Geometry: final body of the model. Coordinates: model frame, mm. Give positions to 0.01 mm unless a question says otherwise; leave off trailing zeros. Loops run counter-clockwise (first coordinate to the right, second up) from the corner with the lowest first, then second, coordinate; pieces in that order, holes last.
from build123d import *

# Parameters (mm, degrees)
F0_W     = 3.175
F0_H     = 17.78
F0_R     = 1.984375
F1_DEPTH = 3.175


with BuildPart() as f1:
    # F0 (on Front) → F1 (new body)
    with BuildSketch(Plane.XZ):
        Polygon((-88.646, -65.532), (-50.546, -65.532), (-50.546, -62.23), (-19.05, -62.23), (-19.05, -65.532), (19.05, -65.532), (19.05, -62.23), (50.546, -62.23), (50.546, -65.532), (88.646, -65.532), (88.646, -62.23), (107.696, -62.23), (196.85, -62.23), (196.85, -44.45), (193.675, -44.45), (193.675, -26.67), (196.85, -26.67), (196.85, -8.89), (193.675, -8.89), (193.675, 8.89), (196.85, 8.89), (196.85, 26.67), (193.675, 26.67), (193.675, 44.45), (196.85, 44.45), (196.85, 62.23), (107.696, 62.23), (88.646, 62.23), (88.646, 65.532), (50.546, 65.532), (50.546, 62.23), (19.05, 62.23), (19.05, 65.532), (-19.05, 65.532), (-19.05, 62.23), (-50.546, 62.23), (-50.546, 65.532), (-88.646, 65.532), (-88.646, 62.23), (-107.696, 62.23), (-196.85, 62.23), (-196.85, 44.45), (-193.675, 44.45), (-193.675, 26.67), (-196.85, 26.67), (-196.85, 8.89), (-193.675, 8.89), (-193.675, -8.89), (-196.85, -8.89), (-196.85, -26.67), (-193.675, -26.67), (-193.675, -44.45), (-196.85, -44.45), (-196.85, -62.23), (-107.696, -62.23), (-88.646, -62.23), align=None)
        with Locations((-106.1085, -35.56)):
            Rectangle(F0_W, F0_H, mode=Mode.SUBTRACT)
        with Locations((-79.121, -52.705)):
            Circle(F0_R, mode=Mode.SUBTRACT)
        with Locations((-66.421, -52.705)):
            Circle(F0_R, mode=Mode.SUBTRACT)
        with Locations((-79.121, -40.005)):
            Circle(F0_R, mode=Mode.SUBTRACT)
        with Locations((-90.2335, -35.56)):
            Rectangle(F0_W, F0_H, mode=Mode.SUBTRACT)
        with Locations((-66.421, -40.005)):
            Circle(F0_R, mode=Mode.SUBTRACT)
        with Locations((66.421, -52.705)):
            Circle(F0_R, mode=Mode.SUBTRACT)
        with Locations((79.121, -52.705)):
            Circle(F0_R, mode=Mode.SUBTRACT)
        with Locations((66.421, -40.005)):
            Circle(F0_R, mode=Mode.SUBTRACT)
        with Locations((79.121, -40.005)):
            Circle(F0_R, mode=Mode.SUBTRACT)
        with Locations((90.2335, -35.56)):
            Rectangle(F0_W, F0_H, mode=Mode.SUBTRACT)
        with Locations((106.1085, -35.56)):
            Rectangle(F0_W, F0_H, mode=Mode.SUBTRACT)
        with Locations((-106.1085, 0)):
            Rectangle(F0_W, F0_H, mode=Mode.SUBTRACT)
        with Locations((-90.2335, 0)):
            Rectangle(F0_W, F0_H, mode=Mode.SUBTRACT)
        with Locations((-106.1085, 35.56)):
            Rectangle(F0_W, F0_H, mode=Mode.SUBTRACT)
        with Locations((-90.2335, 35.56)):
            Rectangle(F0_W, F0_H, mode=Mode.SUBTRACT)
        with Locations((90.2335, 0)):
            Rectangle(F0_W, F0_H, mode=Mode.SUBTRACT)
        with Locations((106.1085, 0)):
            Rectangle(F0_W, F0_H, mode=Mode.SUBTRACT)
        with Locations((90.2335, 35.56)):
            Rectangle(F0_W, F0_H, mode=Mode.SUBTRACT)
        with Locations((106.1085, 35.56)):
            Rectangle(F0_W, F0_H, mode=Mode.SUBTRACT)
    extrude(amount=F1_DEPTH)


solid = f1.part
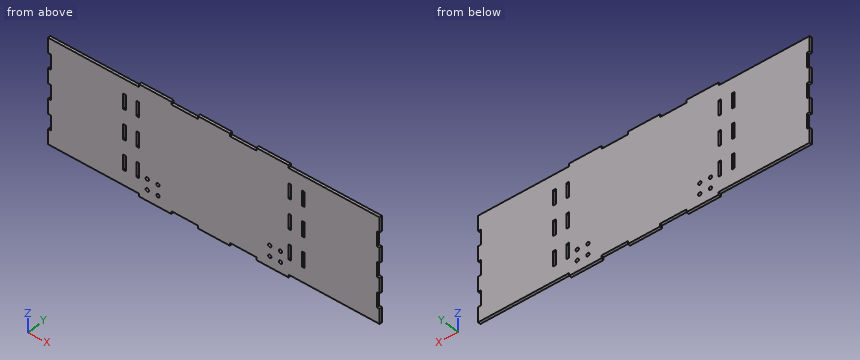
Item 1: Ray query, probe 1 along X at (y, z) = (-2.6, -5.5) (3 decimals); probe 2 along X at (y, z) = (-0.35, -54); probe 3 along Z at (x, y) = (-143.5, -0.2). Return the intervals inside material, ascending.
Values follow:
probe 1: x = -193.675 to -107.696, -104.521 to -91.821, -88.646 to 88.646, 91.821 to 104.521, 107.696 to 193.675
probe 2: x = -196.85 to -80.62, -77.62 to -67.92, -64.92 to 64.92, 67.92 to 77.62, 80.62 to 196.85
probe 3: z = -62.23 to 62.23
Item 2: Section query A-A on z = -1. Return loops of the section in (x, y) (3 decimals).
Values follow:
outline: (-193.675, -3.175) - (-107.696, -3.175) - (-107.696, 0) - (-193.675, 0) - close; (-104.521, -3.175) - (-91.821, -3.175) - (-91.821, 0) - (-104.521, 0) - close; (-88.646, -3.175) - (88.646, -3.175) - (88.646, 0) - (-88.646, 0) - close; (91.821, -3.175) - (104.521, -3.175) - (104.521, 0) - (91.821, 0) - close; (107.696, -3.175) - (193.675, -3.175) - (193.675, 0) - (107.696, 0) - close
Item 3: Section query C-C on y = -0.65. Give the number of separate pieces and of enclosed holes in the cut face, plus the area to 3 significant figures.
Values follow:
separate pieces: 1
enclosed holes: 20
area: 48,600 mm2
Item 4: Section query B-B on x = 28. Return loops of the section in (y, z) (3 decimals), plus the area to 3 significant figures.
Values follow:
outline: (-3.175, -62.23) - (0, -62.23) - (0, 62.23) - (-3.175, 62.23) - close
area: 395 mm2
Item 5: Pin query (flat end, axial travel): pin 1 (1 mm diameter, centred on x = 106, y = -1, fed in from -Z); pin 2 (1.5 mm diameter, centred on y = -2.5, z = 27.5, fed in from -X) (3 decimals); pin 3 (1 mm diameter, centred on y = -2, z = -37.5, fed in from +X) (3 decimals); pin 4 (3 mm diameter, centred on x = 66.421, z = -52.705, fed in from -Y). Return the tip coordinate at first contact, or that it passes through.
Values follow:
pin 1: stops at z = -62.23
pin 2: stops at x = -193.675
pin 3: stops at x = 193.675
pin 4: passes through
